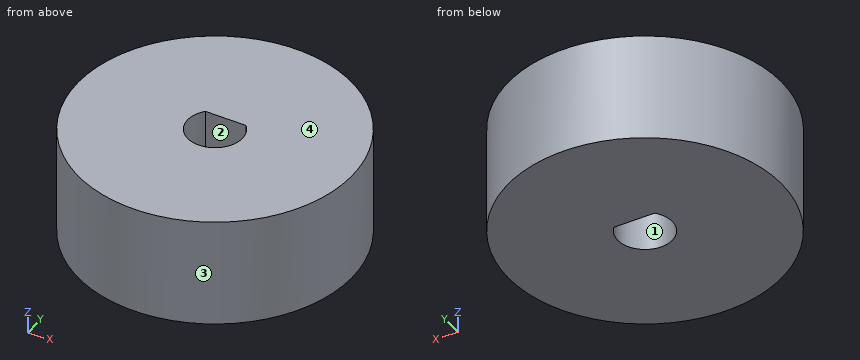
```python
from build123d import *

# Parameters (mm, degrees)
SKETCH1_R                       = 7.5
SKETCH1_R_2                     = 2.5
BOSS_EXTRUDE2_DEPTH             = 2.98
BOSS_EXTRUDE3_REACH             = 4.98
SKETCH1_5_R                     = 2.5
BOSS_EXTRUDE3_DIRECTION_2_REACH = 4.98


with BuildPart() as part:
    # Sketch1 → Boss-Extrude2 (new body, symmetric)
    with BuildSketch(Plane.XY):
        Circle(SKETCH1_R)
        Circle(SKETCH1_R_2, mode=Mode.SUBTRACT)
    extrude(amount=BOSS_EXTRUDE2_DEPTH, both=True)

    # Boss-Extrude3: up to this face of the body (flat: up to its plane)
    boss_extrude3_end = Plane(part.part.faces().sort_by_distance((-7.287867966, 0, 2.98))[0])
    # Sketch1_5 → Boss-Extrude3 (add, up to the picked face)
    with BuildSketch(Plane.XY, mode=Mode.PRIVATE) as boss_extrude3_sk1:
        Circle(SKETCH1_5_R)
        with BuildLine():
            ThreePointArc((-1.118033989, 1), (0, -1.5), (1.118033989, 1))
            Line((1.118033989, 1), (-1.118033989, 1))
        make_face(mode=Mode.SUBTRACT)
    boss_extrude3_tool1 = split(extrude(boss_extrude3_sk1.sketch, amount=BOSS_EXTRUDE3_REACH, mode=Mode.PRIVATE), bisect_by=boss_extrude3_end, keep=Keep.BOTH, mode=Mode.PRIVATE)
    add(boss_extrude3_tool1.solids().sort_by_distance((-2.429289, 0, 0))[0])

    # Boss-Extrude3 direction 2: up to this face of the body (flat: up to its plane)
    boss_extrude3_direction_2_end = Plane(part.part.faces().sort_by_distance((-7.287867966, 0, -2.98))[0])
    # Sketch1_5 → Boss-Extrude3 direction 2 (add, up to the picked face)
    with BuildSketch(Plane.XY, mode=Mode.PRIVATE) as boss_extrude3_direction_2_sk1:
        Circle(SKETCH1_5_R)
        with BuildLine():
            ThreePointArc((-1.118033989, 1), (0, -1.5), (1.118033989, 1))
            Line((1.118033989, 1), (-1.118033989, 1))
        make_face(mode=Mode.SUBTRACT)
    boss_extrude3_direction_2_tool1 = split(extrude(boss_extrude3_direction_2_sk1.sketch, amount=-BOSS_EXTRUDE3_DIRECTION_2_REACH, mode=Mode.PRIVATE), bisect_by=boss_extrude3_direction_2_end, keep=Keep.BOTH, mode=Mode.PRIVATE)
    add(boss_extrude3_direction_2_tool1.solids().sort_by_distance((-2.429289, 0, 0))[0])


solid = part.part
```
Model file for the job. Use its own axes, mm. Face numbers are marked on the shaded views. Give positions to 0.01 mm unless a question says otherwise; leave off trailing zeros. Loops run counter-clockwise (first coordinate to the right, second up) from the corner with the lowest first, then second, coordinate; pieces in that order, holes last. Notation, with made-up numbers: M -18,-14.5 L -3,-14.5 A23 ccw -3,19.5 Z; hole C -32,19 d1. An arc over 180 degrees is marked long. Use one line per item in the form item = value.
Item 1: Slice it at C-C on z = -0.05. List the corners of the cut face in (x, y), and give its area (3 significant figures).
Filled in:
outline = C 0,0 d15; hole M -1.12,1 A1.5 ccw long 1.12,1 Z
area = 170 mm^2
Item 2: Drill centre lines: L1, parallel to Y at x = 0, z = 1.45; L2, parallel to X at y = -0.75, z = -1.95; L3, parallel to Y at x = -3, z = -0.05. Where is each one in solid material? Low to high.
Filled in:
L1 = -7.5 to -1.5, 1 to 7.5
L2 = -7.46 to -1.3, 1.3 to 7.46
L3 = -6.87 to 6.87
Item 3: Slice it at A-A on y = 0. List the corners of the cut face in (x, z), and give its area (3 significant figures).
Filled in:
outline = M -7.5,-2.98 L -1.5,-2.98 L -1.5,2.98 L -7.5,2.98 Z; M 1.5,-2.98 L 7.5,-2.98 L 7.5,2.98 L 1.5,2.98 Z
area = 71.5 mm^2
Item 4: Two-plate mould, pull along Y, no slides. Class the marked faces 1, 2, 3 and 4: released by +Y, released by -Y, zero draft, split by the parting line, or undercut.
Filled in:
face_1 = undercut
face_2 = undercut
face_3 = split by the parting line
face_4 = zero draft
Item 5: Slice it at D-D on x = 6. List the corners of the cut face in (y, z).
Filled in:
outline = M -4.5,-2.98 L 4.5,-2.98 L 4.5,2.98 L -4.5,2.98 Z
Item 6: Slice it at B-B on x = 0. List the corners of the cut face in (y, z), and give its area (3 significant figures).
Filled in:
outline = M -7.5,-2.98 L -1.5,-2.98 L -1.5,2.98 L -7.5,2.98 Z; M 1,-2.98 L 7.5,-2.98 L 7.5,2.98 L 1,2.98 Z
area = 74.5 mm^2
Item 7: Flat gauge pins, fed straight in: pin 1 Ø3 at (x, z) = (1.5, -1.5) entering from +Y; pin 2 Ø1 at (y, z) = (-4.5, 0) entering from -X. Where does each tip first touch, or does it go through?
Filled in:
pin_1 = 7.5
pin_2 = -6.34
